Here's the drawing with two shaded views (mm, measured from the low corner). I have some questions. A direction names the side the tool comes from. Round coordinates to 2 decimals unless told otherwise and drop trailing zeros. Write each loop counter-clockwise with the first axis right and the second up, starting at its lowest first coordinate (ties: lowest second). Pieces come first, ordered by that corner, then holes.
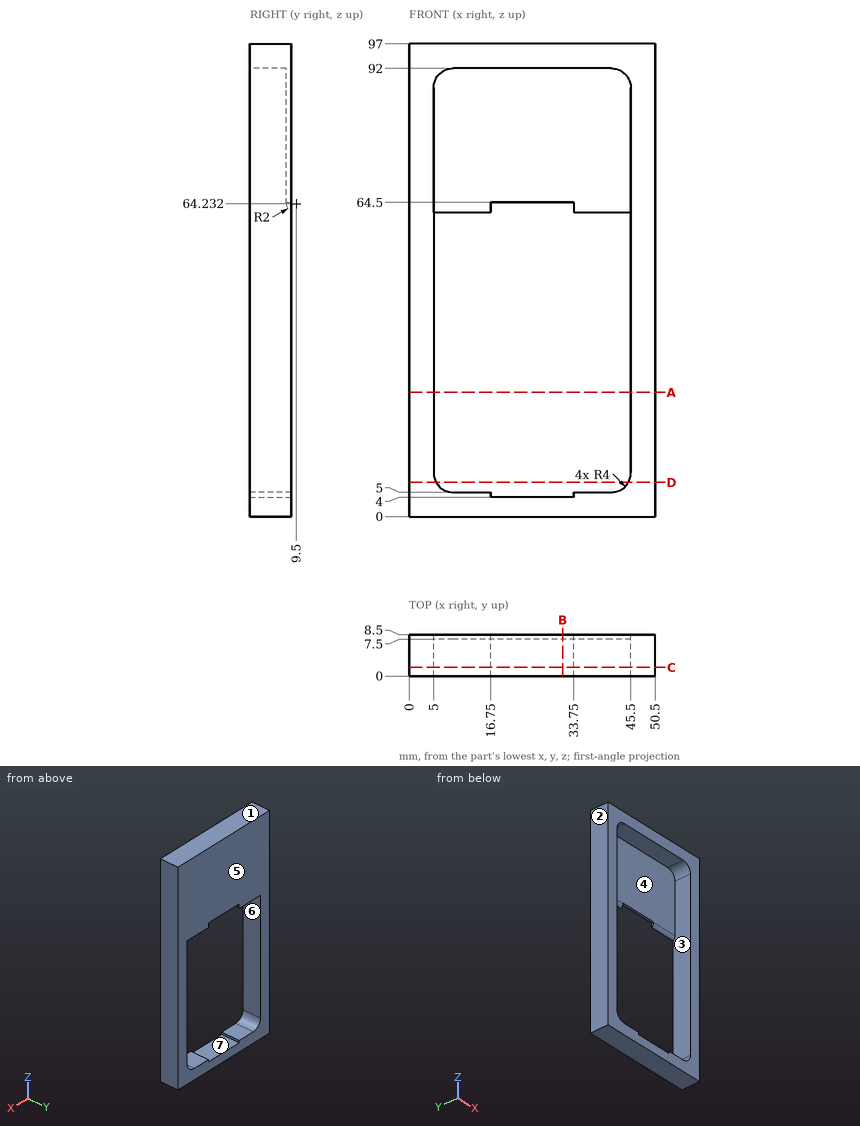
Q1. Imagine slicing it at C-C, the plane y = 1.75. Write out the boundary of the cut face in (x, z).
Q2. We'd pull the mould along X, two halves only. Please class the marked faces 1, 2, 3 and 4: pulls with the +X half, pulls with the -X half, needs draft (parallel to the pull), parting line crosses it, or undercut.
Q3. Imagine slicing it at D-D, the plane z = 7. Write out the boundary of the cut face in (x, y).
Q4. Imagine slicing it at B-B, the plane x = 31.5. Write out the boundary of the cut face in (y, z), then the cut area to 3 significant figures.
Q5. I'm going to push flat-ended pins straight in: pin 1 Ø1.1 at (y, z) = (3.5, 4.5) entering from -X; pin 2 Ø22 at (x, z) = (34, 73) entering from -Y. Where does each tip first touch, or does it pass through?
Q6. If I drill on L1, parallel to X at y = 6.5, z = 39; L2, parallel to Z at x = 28.5, y = 6.25; L3, parallel to Z at x = 38.5, y = 3.75, over which ranges is the centre line in solid material (lowest first)?
Q7. On a 3-axis mill with a long thin cutter (end or side, diameter ignored), from which of +Z, -Z, +X, -X, +Y, -Y can I reach the whole of each face in a straight line? I mean the marked faces 5, 6 and 7. Say none if no direction works.
Q8. Imagine slicing it at A-A, the plane z = 25.5. Write out the boundary of the cut face in (x, y).
Results found:
1. outline: (0, 0) - (50.5, 0) - (50.5, 97) - (0, 97) - close; hole (5, 9) arc R4 ccw to (9, 5) - (16.75, 5) - (16.75, 4) - (33.75, 4) - (33.75, 5) - (41.5, 5) arc R4 ccw to (45.5, 9) - (45.5, 88) arc R4 ccw to (41.5, 92) - (9, 92) arc R4 ccw to (5, 88) - close
2. face 1: needs draft
2. face 2: pulls with the -X half
2. face 3: undercut
2. face 4: undercut
3. outline: (0, 0) - (5.54, 0) - (5.54, 8.5) - (0, 8.5) - close; (44.96, 0) - (50.5, 0) - (50.5, 8.5) - (44.96, 8.5) - close
4. outline: (0, 0) - (8.5, 0) - (8.5, 4) - (0, 4) - close; (0, 92) - (7.5, 92) - (7.5, 64.5) - (8.5, 64.5) - (8.5, 97) - (0, 97) - close
4. area: 104 mm2
5. pin 1: stops at x = 0
5. pin 2: stops at y = 7.5
6. L1: x = 0 to 5, 45.5 to 50.5
6. L2: z = 0 to 4, 92 to 97
6. L3: z = 0 to 5, 92 to 97
7. face 5: +Z, -Z, +X, -X, +Y
7. face 6: -Y
7. face 7: +Y, -Y
8. outline: (0, 0) - (5, 0) - (5, 8.5) - (0, 8.5) - close; (45.5, 0) - (50.5, 0) - (50.5, 8.5) - (45.5, 8.5) - close
